```python
from build123d import *

# Parameters (mm, degrees)
EXTRUDE_1_DEPTH     = 10
SKETCH_2_R          = 40
CUT_EXTRUDE_1_DEPTH = 5


with BuildPart() as part:
    # Эскиз1 → Бобышка-Вытянуть1 (new body)
    with BuildSketch(Plane(origin=(0, 0, 0), x_dir=(1, 0, 0), z_dir=(0, 1, 0))):
        Polygon((1300, 0), (1500, 0), (1500, 800), (500, 800), (500, 300), align=None)
    extrude(amount=EXTRUDE_1_DEPTH)

    # Эскиз2 → Вырез-Вытянуть1 (cut)
    with BuildSketch(Plane.XZ):
        with Locations(Location((1400, -120, 0), (0, 0, 270))):
            Circle(SKETCH_2_R)
        with Locations(Location((1400, -700, 0), (0, 0, 270))):
            Circle(SKETCH_2_R)
    extrude(amount=-CUT_EXTRUDE_1_DEPTH, mode=Mode.SUBTRACT)


solid = part.part
```
Input: part model. Units: mm. Frame: model coordinates. A direction names the side the tool comes from. Coordinates: 2 decimals unless noted, no trailing zeros. Write each loop counter-clockwise with the first axis right and the second up, starting at its lowest first coordinate (ties: lowest second). Pieces come first, ordered by that corner, then holes. Notation, with made-up numbers: (3, 66.25) -> (57, 66.25) arc R30 cw to (57, 98.25) -> close; hole circle Ø9 at (35.25, -24.5). An arc over 180 degrees is marked (long way). Write each question's results on one line, items separated by ' | '.
Item 1: Set-up query: faces 1 (the flat face through (993, 10, -494)), 2 (the flat face through (1401, 5, -119)). Return all of +Z, -Z, +X, -X, +Y, -Y with unobstructed straight access to the full face (end or side cutting, diameter ignored); none if empty.
Conclusion:
face 1: +Z, -Z, +X, -X, +Y | face 2: -Y
Item 2: Mould query, pull axis Z, two halves, no side actions, for faces 3 (the flat face through (894.4, 4.9, -152.1)), 4 (the flat face through (1401, 5, -699)), 5 (the flat face through (993, 0, -494)). Classes: +Z half, -Z half, draft (parallel to the pull), parting line (faces both ways), or undercut.
Conclusion:
face 3: +Z half | face 4: undercut | face 5: draft
Item 3: Pin query (flat end, axial travel): pin 1 Ø10 at (x, z) = (679.5, -434.5) entering from -Y; pin 2 Ø24 at (x, z) = (1391, -697) entering from -Y. Return the tip coordinate at first contact, or that it passes through.
Conclusion:
pin 1: stops at y = 0 | pin 2: stops at y = 5
Item 4: Material intervals for probe 1 along X at (y, z) = (2.5, -700); probe 2 along Z at (x, y) = (619, 0.75) (3 decimals); probe 3 along X at (y, z) = (0.75, -687), sorted ascending.
Conclusion:
probe 1: x = 500 to 1360, 1440 to 1500 | probe 2: z = -800 to -255.375 | probe 3: x = 500 to 1362.17, 1437.83 to 1500
Item 5: Section query A-A on z = -120. Return loops of the section in (x, y).
Conclusion:
outline: (980, 0) -> (1360, 0) -> (1360, 5) -> (1440, 5) -> (1440, 0) -> (1500, 0) -> (1500, 10) -> (980, 10) -> close
Item 6: Section query D-D on z = -700. Return loops of the section in (x, y).
Conclusion:
outline: (500, 0) -> (1360, 0) -> (1360, 5) -> (1440, 5) -> (1440, 0) -> (1500, 0) -> (1500, 10) -> (500, 10) -> close
Item 7: Section query B-B on y = 3.5. Return loops of the section in (x, z), plus the area to 3 significant figures.
Conclusion:
outline: (500, -800) -> (1500, -800) -> (1500, 0) -> (1300, 0) -> (500, -300) -> close; hole circle Ø80 at (1400, -700); hole circle Ø80 at (1400, -120) | area: 670,000 mm^2
Item 8: Section query C-C on x = 1400. Return loops of the section in (y, z), plus the area to 3 significant figures.
Conclusion:
outline: (0, -800) -> (10, -800) -> (10, 0) -> (0, 0) -> (0, -80) -> (5, -80) -> (5, -160) -> (0, -160) -> (0, -660) -> (5, -660) -> (5, -740) -> (0, -740) -> close | area: 7,200 mm^2
